```python
from build123d import *

# Parameters (mm, degrees)
SKETCH1_R           = 2.75
SKETCH1_R_2         = 1.5
BOSS_EXTRUDE2_DEPTH = 1.8
FILLET1_R           = 0.1
CHAMFER1_SIZE       = 0.1


with BuildPart() as part:
    # Sketch1 → Boss-Extrude2 (new body)
    # profile 1 of 7: a face of its own
    with BuildSketch(Plane(origin=(0, 0, 0), x_dir=(1, 0, 0), z_dir=(0, 1, 0))):
        with BuildLine():
            Line((0, 2.75), (-1.58771324, 2.75))
            Line((-1.58771324, 2.75), (-2.381569814, 1.37500008))
            ThreePointArc((-2.381569814, 1.37500008), (-1.37499996, 2.381569884), (0, 2.75))
        make_face()
    # profile 2 of 7: a face of its own
    with BuildSketch(Plane(origin=(0, 0, 0), x_dir=(1, 0, 0), z_dir=(0, 1, 0))):
        with BuildLine():
            ThreePointArc((-2.381569844, -1.375000029), (-2.75, 3e-08), (-2.381569814, 1.37500008))
            Line((-2.381569814, 1.37500008), (-3.175426481, 0))
            Line((-3.175426481, 0), (-2.381569844, -1.375000029))
        make_face()
    # profile 3 of 7: a face of its own
    with BuildSketch(Plane(origin=(0, 0, 0), x_dir=(1, 0, 0), z_dir=(0, 1, 0))):
        with BuildLine():
            Line((1.58771324, 2.75), (0, 2.75))
            ThreePointArc((0, 2.75), (1.374999954, 2.381569887), (2.381569807, 1.375000092))
            Line((2.381569807, 1.375000092), (1.58771324, 2.75))
        make_face()
    # profile 4 of 7: a face of its own
    with BuildSketch(Plane(origin=(0, 0, 0), x_dir=(1, 0, 0), z_dir=(0, 1, 0))):
        with BuildLine():
            Line((3.175426481, 0), (2.381569807, 1.375000092))
            ThreePointArc((2.381569807, 1.375000092), (2.656296008, 0.711752426), (2.75, 0))
            ThreePointArc((2.75, 0), (2.65629601, -0.711752419), (2.381569814, -1.37500008))
            Line((2.381569814, -1.37500008), (3.175426481, 0))
        make_face()
    # profile 5 of 7: a face of its own
    with BuildSketch(Plane(origin=(0, 0, 0), x_dir=(1, 0, 0), z_dir=(0, 1, 0))):
        with BuildLine():
            ThreePointArc((0, -2.75), (-1.374999986, -2.381569869), (-2.381569844, -1.375000029))
            Line((-2.381569844, -1.375000029), (-1.58771324, -2.75))
            Line((-1.58771324, -2.75), (0, -2.75))
        make_face()
    # profile 6 of 7: a face of its own
    with BuildSketch(Plane(origin=(0, 0, 0), x_dir=(1, 0, 0), z_dir=(0, 1, 0))):
        with BuildLine():
            ThreePointArc((2.381569814, -1.37500008), (1.37499996, -2.381569884), (0, -2.75))
            Line((0, -2.75), (1.58771324, -2.75))
            Line((1.58771324, -2.75), (2.381569814, -1.37500008))
        make_face()
    # profile 7 of 7: a face of its own
    with BuildSketch(Plane(origin=(0, 0, 0), x_dir=(1, 0, 0), z_dir=(0, 1, 0))):
        Circle(SKETCH1_R)
        with Locations(Location((0, 0, 0), (0, 0, 270))):
            Circle(SKETCH1_R_2, mode=Mode.SUBTRACT)
    extrude(amount=BOSS_EXTRUDE2_DEPTH)

    # Fillet1
    fillet1_edges = [part.edges().sort_by_distance(p)[0] for p in [
        (2.38156986, 0, -1.375),
        (2.38156986, 0, 1.375),
        (0, 0, 2.75),
        (-2.38156986, 1.8, 1.375),
        (-2.38156986, 0, 1.375),
        (-2.38156986, 0, -1.375),
        (-1.58771324, 0.9, -2.75),
        (1.58771324, 0.9, -2.75),
        (3.175426481, 0.9, 0),
        (1.58771324, 0.9, 2.75),
        (-1.58771324, 0.9, 2.75),
        (-3.175426481, 0.9, 0),
        (2.38156986, 1.8, 1.375),
        (2.38156986, 1.8, -1.375),
        (0, 1.8, -2.75),
        (-2.38156986, 1.8, -1.375),
        (0, 0, -2.75),
    ]]
    fillet(fillet1_edges, radius=FILLET1_R)

    # Chamfer1
    chamfer1_edges = [part.edges().sort_by_distance(p)[0] for p in [
        (0, 1.8, -1.5),
        (0, 0, -1.5),
    ]]
    chamfer(chamfer1_edges, length=CHAMFER1_SIZE)


solid = part.part
```
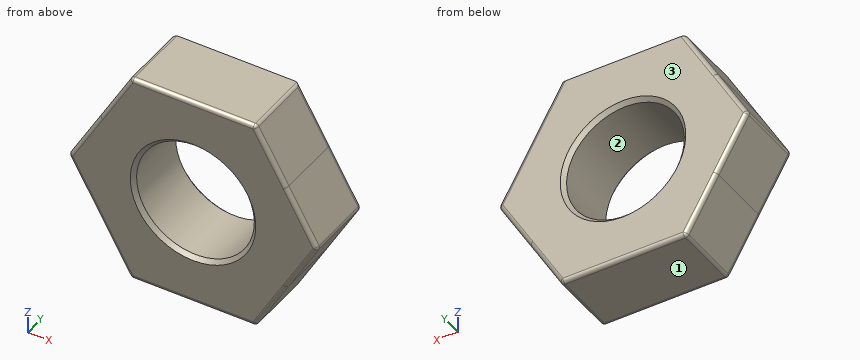
Here's how the part is built. I have some questions about the finished solid (model axes, mm). Face numbers are marked on the shaded views. Round coordinates to 2 decimals unless told otherwise and drop trailing zeros. Loops run counter-clockwise (first coordinate to the right, second up) from the corner with the lowest first, then second, coordinate; pieces in that order, holes last. Notation, with made-up numbers: (-28.5, -21.75) -> (-16.5, -21.75) arc R10 ccw to (-16.5, -11.75) -> close; hole circle Ø2 at (40, 57.5). An arc over 180 degrees is marked (long way). Answer as CSV lines item,"result". Start each with the question number.
1. Imagine slicing it at A-A on y = 1. Write out the boundary of the cut face in (x, z) (3 decimals).
2. Imagine slicing it at B-B on x = 0. Write out the boundary of the cut face in (y, z).
3. I need wall thicknesses on probe 1 along X at (y, z) = (0.65, 0); probe 2 along X at (y, z) = (1.5, -0.3); probe 3 along Z at (x, y) = (1, 1.3). Which ranges of each line are inside material? Lowest first, please. Write a range as from..to.
4. If we mould it in two halves opening along Z, with no side actions, what happens to the marked faces 1, 2 and 3? For each: pulls with the +Z half, pulls with the -Z half, needs draft (parallel to the pull), parting line crosses it, or undercut.
5. I'm going to push a flat-ended pin straight in: P1, Ø1, axis at y = 1.5, z = 1, coming from the +X side. Where does the tip first touch, or does it pass through?
Solution:
1,outline,"(-3.147, -0.05) -> (-1.617, -2.7) arc R0.1 ccw to (-1.53, -2.75) -> (1.53, -2.75) arc R0.1 ccw to (1.617, -2.7) -> (3.147, -0.05) arc R0.1 ccw to (3.147, 0.05) -> (1.617, 2.7) arc R0.1 ccw to (1.53, 2.75) -> (-1.53, 2.75) arc R0.1 ccw to (-1.617, 2.7) -> (-3.147, 0.05) arc R0.1 ccw to start; hole circle Ø3 at (0, 0)"
2,outline,"(0, -2.65) arc R0.1 ccw to (0.1, -2.75) -> (1.7, -2.75) arc R0.1 ccw to (1.8, -2.65) -> (1.8, -1.6) -> (1.7, -1.5) -> (0.1, -1.5) -> (0, -1.6) -> close; (0, 1.6) -> (0.1, 1.5) -> (1.7, 1.5) -> (1.8, 1.6) -> (1.8, 2.75) -> (0.1, 2.75) arc R0.1 ccw to (0, 2.65) -> close"
3,probe 1,"-3.16..-1.5, 1.5..3.16"
3,probe 2,"-3..-1.47, 1.47..3"
3,probe 3,"-2.75..-1.12, 1.12..2.75"
4,face 1,"pulls with the -Z half"
4,face 2,"undercut"
4,face 3,"needs draft"
5,P1,"x = 2.89"
